```python
from build123d import *

# Parameters (mm, degrees)
EXTRUDE_1_DEPTH     = 20
SKETCH_2_R          = 2
SKETCH_2_R_2        = 2.75
CUT_EXTRUDE_1_DEPTH = 75.833147735
EXTRUDE_START       = -35
SKETCH_3_R          = 2
EXTRUDE_2_DEPTH     = 35
SKETCH_4_W          = 7
SKETCH_4_H          = 20
EXTRUDE_3_DEPTH     = 10
FILLET_2_R          = 1
CUT_EXTRUDE_2_DEPTH = 71


with BuildPart() as part:
    # ｽｹｯﾁ1 → ﾎﾞｽ - 押し出し1 (new body)
    with BuildSketch(Plane.XY):
        Polygon((0, 0), (45, 0), (51, 30), (60, 30), (60, -10), (0, -10), align=None)
    extrude(amount=EXTRUDE_1_DEPTH)

    # ｽｹｯﾁ2 → ｶｯﾄ - 押し出し1 (cut, through all)
    with BuildSketch(Plane(origin=(0, 30, 0), x_dir=(1, 0, 0), z_dir=(0, 1, 0))):
        with Locations(Location((55, -10, 0), (0, 0, 270))):
            Circle(SKETCH_2_R)
        with Locations(Location((3, -10, 0), (0, 0, 270))):
            Circle(SKETCH_2_R_2)
    extrude(amount=-CUT_EXTRUDE_1_DEPTH, mode=Mode.SUBTRACT)

    # ｽｹｯﾁ3 → ﾎﾞｽ - 押し出し2 (add)
    with BuildSketch(Plane.XZ.offset(10).offset(EXTRUDE_START)):
        with Locations(Location((55, 10, 0), (0, 0, 90))):
            Circle(SKETCH_3_R)
    extrude(amount=EXTRUDE_2_DEPTH)

    # ｽｹｯﾁ4 → ﾎﾞｽ - 押し出し3 (add)
    with BuildSketch(Plane(origin=(0, 0, 0), x_dir=(1, 0, 0), z_dir=(0, 1, 0))):
        with Locations((-3.5, -10)):
            Rectangle(SKETCH_4_W, SKETCH_4_H)
    extrude(amount=-EXTRUDE_3_DEPTH)

    # ﾌｨﾚｯﾄ2
    fillet_2_edges = [part.edges().sort_by_distance(p)[0] for p in [
        (60, 10, 20),
        (48, 15, 20),
        (-7, -5, 20),
        (-7, -5, 0),
        (48, 15, 0),
        (60, 10, 0),
    ]]
    fillet(fillet_2_edges, radius=FILLET_2_R)

    # ｽｹｯﾁ5 → ｶｯﾄ - 押し出し2 (cut, through all)
    with BuildSketch(Plane(origin=(0, 0, 0), x_dir=(1, 0, 0), z_dir=(0, 1, 0))):
        with BuildLine():
            Line((-2, -7.25), (40, -7.25))
            ThreePointArc((40, -7.25), (42.75, -10), (40, -12.75))
            Line((40, -12.75), (-2, -12.75))
            ThreePointArc((-2, -12.75), (-4.75, -10), (-2, -7.25))
        make_face()
    extrude(amount=-CUT_EXTRUDE_2_DEPTH, mode=Mode.SUBTRACT)


solid = part.part
```
CAD build for the part. Positions are in the model's coordinates, mm. A direction names the side the tool comes from. Coordinates: 2 decimals unless noted, no trailing zeros. Order: outer loops, then holes, each group sorted by start corner. A loop starts at its lowest first (then second) coordinate and runs counter-clockwise, first axis right, second up.
(1) Saw through at C-C, the plane x = 55. Write the cut outline in (y, z), and give its area (3 significant figures).
Solution:
outline: (-10, 0) - (30, 0) - (30, 8) - (25, 8) - (25, 12) - (30, 12) - (30, 20) - (-10, 20) - close
area: 780 mm2
(2) Saw through at D-D, the plane z = 3.75. Write the cut outline in (x, y), and give its area (3 significant figures).
Solution:
outline: (-7, -10) - (60, -10) - (60, 30) - (51, 30) - (45, 0) - (-7, 0) - close
area: 1,030 mm2
(3) Pin check, flat tips, straight feed: pin 1 Ø1 at (x, z) = (27.5, 17) entering from +Y; pin 2 Ø5 at (x, z) = (7.5, 9) entering from -Y. Stop position of each tip, or through.
Solution:
pin 1: stops at y = 0
pin 2: stops at y = -10
(4) Saw through at B-B, the plane x = 8.5. Write the cut outline in (y, z), and give its area (3 significant figures).
Solution:
outline: (-10, 0) - (0, 0) - (0, 7.25) - (-10, 7.25) - close; (-10, 12.75) - (0, 12.75) - (0, 20) - (-10, 20) - close
area: 145 mm2
(5) Which spindle directions (+Z, -Z, +X, -X, +Y, -Y) get a long thin tool onto all of the face, cutting with end or side? Do faces 1 (the face through (57, 28, 10)), 2 (the face through (19, 0, 5)), 3 (the face through (-7, -5, 10)), 4 (the face through (19, -5, 12.75)). Say none if no direction does.
Solution:
face 1: +Y
face 2: +Z, -Z, -X, +Y
face 3: +Z, -Z, -X, +Y, -Y
face 4: +Y, -Y
(6) Saw through at A-A, the plane z = 10. Write the cut outline in (x, y).
Solution:
outline: (-7, -10) - (-4.75, -10) - (-4.75, 0) - (-7, 0) - close; (42.75, -10) - (60, -10) - (60, 30) - (57, 30) - (57, 25) - (53, 25) - (53, 30) - (51, 30) - (45, 0) - (42.75, 0) - close
(7) Mould opens along X. For faces 5 (the face through (48.34, 15.25, 19.7)), 6 (the face through (42.75, -4.93, 9.94)), 7 (the face through (60, 10, 10)), 8 (the face through (55, 25, 10)) say: released by +X, released by -X, zero draft, split by the parting line, or undercut.
Solution:
face 5: released by -X
face 6: undercut
face 7: released by +X
face 8: undercut
(8) Drill centre lines: L1, parallel to Z at x = 55, y = 27; L2, parallel to Y at x = 6, z = 2; L3, parallel to X at y = 27.95, z = 10. Where is each one in solid material? Low to high.
Solution:
L1: z = 0 to 8, 12 to 20
L2: y = -10 to 0
L3: x = 50.59 to 53, 57 to 60
